Build history of the part. All positions in model axes, mm. A direction names the side the tool comes from. Give positions to 0.01 mm unless a question says otherwise; leave off trailing zeros. Loops run counter-clockwise (first coordinate to the right, second up) from the corner with the lowest first, then second, coordinate; pieces in that order, holes last. Notation, with made-up numbers: (22.25, -8) -> (27.25, -8) arc R25 cw to (27.25, 15) -> close; hole circle Ø10 at (-29.5, -19). An arc over 180 degrees is marked (long way). Answer as a JSON object with one key per item and string values. Group by question number.
Q1. Tool access for faces 4 (the flat face through (-47.749, 1.2, 3.5)), 5 (the flat face through (0, -45.749, 3)), 6 (the flat face through (9, -1, 4)): list every direction of +Z, -Z, +X, -X, +Y, -Y with a clear straight run to the whole face (end or side of a thin tool).
Q2. Band-saw the part on C-C, the plane y = -32. Write the cut outline in (x, z).
Q3. Drop flat-ended pins along their axis: pin 1 (4 mm diameter, centred on x = 0.01, y = 9.07, fed in from -Z); pin 2 (1.2 mm diameter, centred on y = 0, z = 3.5, fed in from -X); pin 3 (1.8 mm diameter, centred on x = -31, y = -18, fed in from -Z); pin 4 (12 mm diameter, centred on x = -13, y = 19, fed in from -Z). Give the stop position or say it passes through.
Q4. Band-saw the part on A-A, the plane y = -18. Write the cut outline in (x, z), plus the area to 3 significant figures.
Q5. Two-plate mould, pull along Y, no slides. Class faces 1 (the cylindrical face through (-35.015, 35.693, 3.451)), 2 (the flat face through (-26, -15, 0)), 3 (the cylindrical face through (25.308, -14.547, 1.972)): pulls with the +Y half, pulls with the -Y half, needs draft (parallel to the pull), parting line crosses it, or undercut.
Q6. Wall check: probe 1 along X at (y, z) = (-1, 6); probe 2 along Y at (x, z) = (0, 3); probe 3 along Z at (x, y) = (-45.95, 0). Give the ranges that are in metal, low to high. Write a range as from..to.
Q7. Band-saw the part on B-B, the plane x = -14. Write the cut outline in (y, z), plus the area to 3 significant figures.
from build123d import *

# Parameters (mm, degrees)
F0_R      = 1.5
F1_DEPTH  = 7
F3_DEPTH  = 4
F5_D      = 2
F5_DEPTH  = 4
F5_TIP    = 0.600860619
F7_D      = 2
F7_DEPTH  = 4
F7_TIP    = 0.600860619
F9_DEPTH  = 4
F10_D     = 3
F10_DEPTH = 4
F10_TIP   = 0.9012909285


with BuildPart() as f1:
    # F0 (on Top) → F1 (new body)
    with BuildSketch(Plane.XY):
        with BuildLine():
            ThreePointArc((-5, 49.7493718553), (-35.3553390204, 35.3553390982), (-49.7493718443, 5.0000001095))
            Line((-49.7493718443, 5.0000001095), (-47.7493718443, 5.0000001095))
            Line((-47.7493718443, 5.0000001095), (-47.7493718443, -4.9999998882))
            Line((-47.7493718443, -4.9999998882), (-49.7493718666, -4.9999998882))
            ThreePointArc((-49.7493718666, -4.9999998882), (-35.3553390593, -35.3553390593), (-4.9999998882, -49.7493718666))
            Line((-4.9999998882, -49.7493718666), (-7.4999998882, -45.7493718443))
            Line((-7.4999998882, -45.7493718443), (7.5000001118, -45.7493718443))
            Line((7.5000001118, -45.7493718443), (5.0000001095, -49.7493718443))
            ThreePointArc((5.0000001095, -49.7493718443), (35.355339138, -35.3553389807), (49.7493718666, -4.9999998882))
            Line((49.7493718666, -4.9999998882), (47.7493718666, -4.9999998882))
            Line((47.7493718666, -4.9999998882), (47.7493718443, 5.0000001095))
            Line((47.7493718443, 5.0000001095), (49.7493718443, 5.0000001095))
            ThreePointArc((49.7493718443, 5.0000001095), (35.3553390204, 35.3553390982), (5, 49.7493718553))
            Line((5, 49.7493718553), (7.5, 45.7493718553))
            Line((7.5, 45.7493718553), (-7.5, 45.7493718553))
            Line((-7.5, 45.7493718553), (-5, 49.7493718553))
        make_face()
        with Locations((-30.99729, -18)):
            Circle(F0_R, mode=Mode.SUBTRACT)
        with Locations((30.99729, -18)):
            Circle(F0_R, mode=Mode.SUBTRACT)
        with BuildLine():
            ThreePointArc((-41.8330013267, -7.5), (-42.5, 0), (-41.8330013267, 7.5))
            Line((-41.8330013267, 7.5), (-35.8330013267, 7.5))
            Line((-35.8330013267, 7.5), (-35.8330013267, -7.5))
            Line((-35.8330013267, -7.5), (-41.8330013267, -7.5))
        make_face(mode=Mode.SUBTRACT)
        with Locations((-30.99729, 27.99879)):
            Circle(F0_R, mode=Mode.SUBTRACT)
        with Locations((0, 38)):
            Circle(F0_R, mode=Mode.SUBTRACT)
        with Locations((30.99729, 27.99879)):
            Circle(F0_R, mode=Mode.SUBTRACT)
    extrude(amount=F1_DEPTH)

    # F2 (on face) → F3 (cut)
    with BuildSketch(Plane(origin=(0, 0, 0), x_dir=(1, 0, 0), z_dir=(0, 0, -1))):
        with BuildLine():
            Line((-33.2126875853, 11.7240947344), (-40.0763431849, 14.1469684711))
            ThreePointArc((-40.0763431849, 14.1469684711), (-42.1991788884, -5.0477025611), (-35.6090242019, -23.2001593829))
            ThreePointArc((-35.6090242019, -23.2001593829), (-26.0583647767, -23.5376280677), (-26.6909660756, -33.0732872565))
            ThreePointArc((-26.6909660756, -33.0732872565), (-16.571886566, -39.1359499136), (-5.1761259013, -42.1836191033))
            ThreePointArc((-5.1761259013, -42.1836191033), (0, -31.344555), (5.1761259013, -42.1836191033))
            ThreePointArc((5.1761259013, -42.1836191033), (16.571886566, -39.1359499136), (26.6909660756, -33.0732872565))
            ThreePointArc((26.6909660756, -33.0732872565), (26.0583647767, -23.5376280677), (35.6090242019, -23.2001593829))
            ThreePointArc((35.6090242019, -23.2001593829), (42.1991788884, -5.0477025611), (40.0763431849, 14.1469684711))
            Line((40.0763431849, 14.1469684711), (33.2126875853, 11.7240947344))
            ThreePointArc((33.2126875853, 11.7240947344), (25.241859967, 14.6578452312), (26.6446104223, 23.0347943213))
            Line((26.6446104223, 23.0347943213), (32.150922703, 27.7951105295))
            ThreePointArc((32.150922703, 27.7951105295), (0, 42.5), (-32.150922703, 27.7951105295))
            Line((-32.150922703, 27.7951105295), (-26.6446104223, 23.0347943213))
            ThreePointArc((-26.6446104223, 23.0347943213), (-25.241859967, 14.6578452312), (-33.2126875853, 11.7240947344))
        make_face()
    extrude(amount=-F3_DEPTH, mode=Mode.SUBTRACT)

    # F5
    with Locations(Plane(origin=(-47.7493718443, 0, 0), x_dir=(0, -1, 0), z_dir=(-1, 0, 0))):
        with Locations((-1.106e-07, 3.5)):
            Hole(F5_D / 2, depth=F5_DEPTH)
            with Locations((0, 0, -(F5_DEPTH + F5_TIP / 2))):  # 118° drill point
                Cone(0, F5_D / 2, F5_TIP, mode=Mode.SUBTRACT)

    # F7
    with Locations(Plane(origin=(47.7493718554, 1.062e-07, 0), x_dir=(-2.2e-09, 1, 0), z_dir=(1, 2.2e-09, 0))):
        with Locations((4.4e-09, 3.5)):
            Hole(F7_D / 2, depth=F7_DEPTH)
            with Locations((0, 0, -(F7_DEPTH + F7_TIP / 2))):  # 118° drill point
                Cone(0, F7_D / 2, F7_TIP, mode=Mode.SUBTRACT)

    # F8 (on Top) → F9 (join)
    with BuildSketch(Plane.XY):
        with BuildLine():
            Line((-4.9882119756, 9.0746689573), (-4.9882119756, -9.0608097649))
            ThreePointArc((-4.9882119756, -9.0608097649), (0.0117880244, -14.0608097649), (5.0117880244, -9.0608097649))
            Line((5.0117880244, -9.0608097649), (5.0117880244, 9.0746689573))
            ThreePointArc((5.0117880244, 9.0746689573), (0.0117880244, 14.0746689573), (-4.9882119756, 9.0746689573))
        make_face()
    extrude(amount=F9_DEPTH)

    # F10
    with Locations(Plane(origin=(0, 0, 0), x_dir=(1, 0, 0), z_dir=(0, 0, -1))):
        with Locations((0.0117880244, 9.0608097649), (0.0117880244, -9.0746689573)):
            Hole(F10_D / 2, depth=F10_DEPTH)
            with Locations((0, 0, -(F10_DEPTH + F10_TIP / 2))):  # 118° drill point
                Cone(0, F10_D / 2, F10_TIP, mode=Mode.SUBTRACT)


solid = f1.part
Worked answers:
{
 "1": {"face 4": "+Z, -Z, -X", "face 5": "+Z, -Z", "face 6": "-Z"},
 "2": {"outline": "(-38.42, 0) -> (-27.97, 0) -> (-27.97, 4) -> (27.97, 4) -> (27.97, 0) -> (38.42, 0) -> (38.42, 7) -> (-38.42, 7) -> close"},
 "3": {"pin 1": "z = 0", "pin 2": "x = -43.51", "pin 3": "through", "pin 4": "z = 4"},
 "4": {"outline": "(-46.65, 0) -> (-32.5, 0) -> (-32.5, 7) -> (-46.65, 7) -> close; (-29.5, 0) -> (-24.34, 0) -> (-24.34, 4) -> (24.34, 4) -> (24.34, 0) -> (29.5, 0) -> (29.5, 7) -> (-29.5, 7) -> close; (32.5, 0) -> (46.65, 0) -> (46.65, 7) -> (32.5, 7) -> close", "area": "416 mm2"},
 "5": {"face 1": "pulls with the +Y half", "face 2": "needs draft", "face 3": "undercut"},
 "6": {"probe 1": "-47.75..-42.49, -35.83..47.75", "probe 2": "-45.75..-42.5, -14.06..-10.56, -7.56..7.57, 10.57..14.07, 31.34..36.5, 39.5..45.75", "probe 3": "0..2.5, 4.5..7"},
 "7": {"outline": "(-48, 0) -> (-40.13, 0) -> (-40.13, 4) -> (40.13, 4) -> (40.13, 0) -> (48, 0) -> (48, 7) -> (-48, 7) -> close", "area": "351 mm2"}
}
